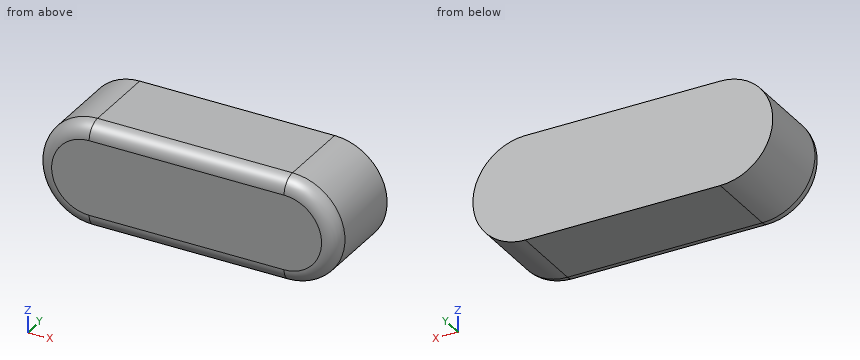
from build123d import *

# Parameters (mm, degrees)
F1_DEPTH = 3
F2_R     = 0.5


with BuildPart() as f1:
    # F0 (on Front) → F1 (new body)
    with BuildSketch(Plane.XZ):
        with BuildLine():
            Line((-3.647967, 1.75), (-10.147967, 1.75))
            ThreePointArc((-10.147967, 1.75), (-11.897967, 0), (-10.147967, -1.75))
            Line((-10.147967, -1.75), (-3.647967, -1.75))
            ThreePointArc((-3.647967, -1.75), (-1.897967, 0), (-3.647967, 1.75))
        make_face()
    extrude(amount=F1_DEPTH)

    # F2
    f2_edges = [f1.edges().sort_by_distance(p)[0] for p in [
        (-6.897967, -3, 1.75),
        (-1.897967, -3, 0),
        (-6.897967, -3, -1.75),
        (-11.897967, -3, 0),
    ]]
    fillet(f2_edges, radius=F2_R)


solid = f1.part
Here's how the part is built. I have some questions about the finished solid (model axes, mm). Give positions to 0.01 mm unless a question says otherwise; leave off trailing zeros. Order: outer loops, then holes, each group sorted by start corner. A loop starts at its lowest first (then second) coordinate and runs counter-clockwise, first axis right, second up. Notation, with made-up numbers: (36, 25) -> (45, 25) arc R30 ccw to (45, 49) -> close; hole circle Ø6 at (44, 21.25). An arc over 180 degrees is marked (long way). One line per item, written item: value. Start each with the question number.
1. Will this pin go through, and if not, where does the flat tip stop? pin 1 Ø1.5 at (y, z) = (-2.5, 1) entering from -X.
2. Imagine slicing it at B-B, the plane y = -0.6. List the corners of the cut face in (x, z) for me.
3. I need wall thicknesses on probe 1 along Y at (x, z) = (-9, 1.3); probe 2 along Z at (x, y) = (-11, -1.55); probe 3 along Z at (x, y) = (-2.25, -1.8). Which ranges of each line are inside material? Lowest first, please. Write a range as from..to.
4. Imagine slicing it at A-A, the plane y = -2.8. List the corners of the cut face in (x, z) for me, plus the area to 3 significant figures.
Values follow:
1. pin 1: stops at x = -11.88
2. outline: (-10.15, -1.75) -> (-3.65, -1.75) arc R1.75 ccw to (-3.65, 1.75) -> (-10.15, 1.75) arc R1.75 ccw to start
3. probe 1: y = -3..0
3. probe 2: z = -1.53..1.53
3. probe 3: z = -1.05..1.05
4. outline: (-10.15, -1.65) -> (-3.65, -1.65) arc R1.65 ccw to (-3.65, 1.65) -> (-10.15, 1.65) arc R1.65 ccw to start
4. area: 30.0 mm2
